```python
from build123d import *

# Parameters (mm, degrees)
SKETCH_1_W          = 60
SKETCH_1_H          = 31
EXTRUDE_1_DEPTH     = 10
CUT_EXTRUDE_1_DEPTH = 10
EXTRUDE_2_DEPTH     = 10
SKETCH_4_R          = 1
CUT_EXTRUDE_2_DEPTH = 10
SKETCH_5_W          = 39
SKETCH_5_H          = 20
SKETCH_5_W_2        = 0.67251462
SKETCH_5_H_2        = 5
SKETCH_5_W_3        = 11
SKETCH_5_H_3        = 2
CUT_EXTRUDE_3_DEPTH = 0.1
SKETCH_6_R          = 4
EXTRUDE_3_DEPTH     = 1.5
SKETCH_7_R          = 2
EXTRUDE_4_DEPTH     = 3


with BuildPart() as part:
    # 草图1 → 凸台-拉伸1 (new body)
    with BuildSketch(Plane(origin=(0, 0, 0), x_dir=(1, 0, 0), z_dir=(0, 1, 0))):
        with Locations((30, 15.5)):
            Rectangle(SKETCH_1_W, SKETCH_1_H)
    extrude(amount=EXTRUDE_1_DEPTH)

    # 草图2 → 切除-拉伸1 (cut)
    with BuildSketch(Plane(origin=(0, 10, 0), x_dir=(1, 0, 0), z_dir=(0, 1, 0))):
        Polygon((14, 0), (14, 1.5), (12.5, 1.5), (12.5, 3), (49.5, 3), (49.5, 2), (47, 2), (49.5, 0), align=None)
        Polygon((0, 30), (5, 31), (0, 31), align=None)
    extrude(amount=-CUT_EXTRUDE_1_DEPTH, mode=Mode.SUBTRACT)

    # 草图3 → 凸台-拉伸2 (add, through all)
    with BuildSketch(Plane(origin=(0, 10, 0), x_dir=(1, 0, 0), z_dir=(0, 1, 0))):
        with BuildLine():
            Line((61, 31), (60, 31))
            Line((60, 31), (60, 25))
            Line((60, 25), (61.7, 25))
            ThreePointArc((61.7, 25), (62.265685425, 25.234314575), (62.5, 25.8))
            Line((62.5, 25.8), (62.5, 28))
            Line((62.5, 28), (61, 31))
        make_face()
        Polygon((36, 31), (60, 31), (60, 32.5), (39.5, 32.5), align=None)
    extrude(amount=-EXTRUDE_2_DEPTH)

    # 草图4 → 切除-拉伸2 (cut)
    with BuildSketch(Plane.ZY):
        with Locations((-18.5, 5)):
            Circle(SKETCH_4_R)
        with Locations((-10.5, 5)):
            Circle(SKETCH_4_R)
    extrude(amount=-CUT_EXTRUDE_2_DEPTH, mode=Mode.SUBTRACT)

    # 草图5 → 切除-拉伸3 (cut)
    # profile 1 of 3: a face of its own
    with BuildSketch(Plane(origin=(0, 10, 0), x_dir=(1, 0, 0), z_dir=(0, 1, 0))):
        with Locations((34, 15)):
            Rectangle(SKETCH_5_W, SKETCH_5_H)
        Polygon((21.962260416, 17.792968637), (21.377465095, 17.792968637), (21.377465095, 21.360220099), (21.318985562, 21.360220099), (20.617231176, 17.792968637), (20.149394919, 17.792968637), (19.447640533, 21.360220099), (19.389161001, 21.360220099), (19.389161001, 17.792968637), (18.804365679, 17.792968637), (18.804365679, 22.792968637), (19.710798428, 22.792968637), (20.354073282, 19.48887507), (20.412552814, 19.48887507), (21.055827668, 22.792968637), (21.962260416, 22.792968637), align=None, mode=Mode.SUBTRACT)
        with Locations((24.111383223, 20.292968637)):
            Rectangle(SKETCH_5_W_2, SKETCH_5_H_2, mode=Mode.SUBTRACT)
        Polygon((29.359921235, 22.237413081), (28.190330592, 22.237413081), (28.190330592, 17.792968637), (27.517815972, 17.792968637), (27.517815972, 22.237413081), (26.348225329, 22.237413081), (26.348225329, 22.792968637), (29.359921235, 22.792968637), align=None, mode=Mode.SUBTRACT)
        with BuildLine():
            Line((33.102611293, 17.734489105), (32.60553527, 17.734489105))
            Line((32.60553527, 17.734489105), (32.517815972, 18.14384583))
            add(Edge.make_bspline(
                [(32.517815972, 18.14384583), (32.496335049, 18.114894908), (32.452578683, 18.05592225), (32.366892397, 17.979393037), (32.266643174, 17.909470256), (32.151128708, 17.848642528), (32.025699097, 17.798099411), (31.892521927, 17.760859691), (31.75360842, 17.739070297), (31.659108429, 17.736026374), (31.611383223, 17.734489105)],
                knots=[0, 0, 0, 0, 0.837184115, 1.705333332, 2.658671207, 3.677307666, 4.736711015, 5.80083511, 6.889358663, 8, 8, 8, 8], degree=3))
            add(Edge.make_bspline(
                [(31.611383223, 17.734489105), (31.560714868, 17.736021013), (31.46008263, 17.739063531), (31.311817937, 17.76762581), (31.16729555, 17.811965229), (31.027834691, 17.8755244), (30.891473719, 17.955281193), (30.760771836, 18.055054478), (30.632955326, 18.171046345), (30.509527994, 18.304333327), (30.396774962, 18.45853747), (30.297519239, 18.634098702), (30.215913122, 18.832381023), (30.147881926, 19.050856514), (30.096694353, 19.291330684), (30.05919444, 19.552513083), (30.036438806, 19.835379254), (30.033799786, 20.03103084), (30.032435855, 20.132149923)],
                knots=[0, 0, 0, 0, 0.758179789, 1.505818141, 2.253143624, 3.017869083, 3.795858856, 4.614441485, 5.475677495, 6.378750386, 7.330399785, 8.330312341, 9.391702904, 10.535751225, 11.753218739, 13.069914954, 14.485637047, 16, 16, 16, 16], degree=3))
            add(Edge.make_bspline(
                [(30.032435855, 20.132149923), (30.033524015, 20.243005064), (30.035631477, 20.457700531), (30.056303392, 20.768942629), (30.090571093, 21.058155718), (30.137547246, 21.32565553), (30.198737704, 21.571304744), (30.274571201, 21.795097166), (30.362412052, 21.997908599), (30.466184437, 22.177806713), (30.5809145, 22.336396595), (30.705728208, 22.474833232), (30.84257532, 22.589830475), (30.987256047, 22.687082934), (31.14384738, 22.76138369), (31.310614479, 22.812780351), (31.487019509, 22.845452192), (31.607987718, 22.849419101), (31.669862755, 22.851448169)],
                knots=[0, 0, 0, 0, 1.495213205, 2.895810661, 4.205263949, 5.422164245, 6.557127206, 7.616570214, 8.606403325, 9.533523062, 10.412081511, 11.242765381, 12.040838916, 12.817408929, 13.588463244, 14.369296309, 15.165897781, 16, 16, 16, 16], degree=3))
            add(Edge.make_bspline(
                [(31.669862755, 22.851448169), (31.724465447, 22.850157263), (31.831330219, 22.847630786), (31.986728106, 22.823055348), (32.133156944, 22.78417248), (32.270367528, 22.72996005), (32.39858198, 22.660001985), (32.517012997, 22.573895908), (32.626334766, 22.471986726), (32.725227795, 22.355220127), (32.813311094, 22.226144327), (32.892302084, 22.088427367), (32.956880517, 21.940329471), (33.009859712, 21.783333409), (33.052602879, 21.617693101), (33.080734277, 21.442188631), (33.100302009, 21.258143875), (33.101830982, 21.132132363), (33.102611293, 21.067822438)],
                knots=[0, 0, 0, 0, 1.017118894, 1.990637724, 2.924249984, 3.836374462, 4.733711419, 5.639510097, 6.558385009, 7.513001497, 8.485403533, 9.467718841, 10.467915617, 11.491402174, 12.553806325, 13.652248568, 14.801825996, 16, 16, 16, 16], degree=3))
            Line((33.102611293, 21.067822438), (32.45933644, 21.067822438))
            add(Edge.make_bspline(
                [(32.45933644, 21.067822438), (32.458729978, 21.117290953), (32.457551218, 21.213441346), (32.448009389, 21.352666796), (32.431312149, 21.482310098), (32.410867073, 21.602817265), (32.380914637, 21.71323506), (32.347227761, 21.814971363), (32.304498884, 21.905966508), (32.256760295, 21.988236327), (32.203036922, 22.060957155), (32.142500003, 22.123391188), (32.077558088, 22.176617179), (32.007055999, 22.22128447), (31.930094878, 22.254334745), (31.84783057, 22.277999378), (31.760739913, 22.29416845), (31.700622449, 22.295309026), (31.669862755, 22.295892614)],
                knots=[0, 0, 0, 0, 1.442265648, 2.803286258, 4.065667754, 5.252751118, 6.363271917, 7.39841691, 8.373155808, 9.288343585, 10.168233039, 11.001900497, 11.817228588, 12.611567034, 13.426963055, 14.24959516, 15.104388078, 16, 16, 16, 16], degree=3))
            add(Edge.make_bspline(
                [(31.669862755, 22.295892614), (31.631828893, 22.294563094), (31.557924625, 22.291979681), (31.450633434, 22.268061012), (31.350844775, 22.23047274), (31.257857421, 22.177333742), (31.172866818, 22.108722655), (31.097286108, 22.023210173), (31.025577535, 21.925676313), (30.964584262, 21.809804655), (30.908423102, 21.678016537), (30.863297772, 21.525387026), (30.821490016, 21.353610633), (30.790614597, 21.160102718), (30.763920798, 20.947080428), (30.748343708, 20.713136474), (30.735099548, 20.458990692), (30.734500993, 20.282340978), (30.734190241, 20.190629456)],
                knots=[0, 0, 0, 0, 0.713867664, 1.387128832, 2.054865043, 2.71116651, 3.391329963, 4.097256694, 4.850367561, 5.660840087, 6.551597142, 7.538616976, 8.647598492, 9.872123473, 11.218389466, 12.680914074, 14.276824714, 16, 16, 16, 16], degree=3))
            add(Edge.make_bspline(
                [(30.734190241, 20.190629456), (30.73483395, 20.103968299), (30.736071349, 19.937379816), (30.750607233, 19.698223249), (30.772176165, 19.47971091), (30.805076542, 19.282835127), (30.843512642, 19.105844287), (30.894744195, 18.950545195), (30.953134814, 18.815066175), (31.022715541, 18.70062504), (31.098039155, 18.604304965), (31.175512101, 18.520836306), (31.255451263, 18.450044406), (31.338684162, 18.392015675), (31.424300922, 18.345320992), (31.514153456, 18.314560623), (31.605733113, 18.293658802), (31.667942985, 18.291250783), (31.699102521, 18.29004466)],
                knots=[0, 0, 0, 0, 1.763137318, 3.38927359, 4.873732177, 6.228632264, 7.449226689, 8.554896297, 9.551299921, 10.444451664, 11.27164773, 12.035603122, 12.759076972, 13.439665674, 14.096862192, 14.735741838, 15.366761318, 16, 16, 16, 16], degree=3))
            add(Edge.make_bspline(
                [(31.699102521, 18.29004466), (31.72983218, 18.290848844), (31.790132284, 18.292426876), (31.878031693, 18.305615952), (31.961197096, 18.327367151), (32.039477559, 18.357607005), (32.112590811, 18.396886673), (32.180290182, 18.444875026), (32.24233728, 18.502053953), (32.300237525, 18.567322721), (32.352177249, 18.64200929), (32.396916088, 18.726819825), (32.434506327, 18.820857568), (32.464574283, 18.924703583), (32.488267476, 19.037669605), (32.505105864, 19.159978961), (32.516471005, 19.291925027), (32.517356401, 19.383080592), (32.517815972, 19.430395538)],
                knots=[0, 0, 0, 0, 0.926763241, 1.818566216, 2.674466499, 3.515830513, 4.344194496, 5.172200422, 6.012506428, 6.88440238, 7.799833367, 8.749917039, 9.771239203, 10.849892544, 12.007626437, 13.250589984, 14.572899121, 16, 16, 16, 16], degree=3))
            Line((32.517815972, 19.430395538), (32.517815972, 19.752032964))
            Line((32.517815972, 19.752032964), (31.611383223, 19.752032964))
            Line((31.611383223, 19.752032964), (31.611383223, 20.30758852))
            Line((31.611383223, 20.30758852), (33.102611293, 20.30758852))
            Line((33.102611293, 20.30758852), (33.102611293, 17.734489105))
        make_face(mode=Mode.SUBTRACT)
    # profile 2 of 3: a face of its own
    with BuildSketch(Plane(origin=(0, 10, 0), x_dir=(1, 0, 0), z_dir=(0, 1, 0))):
        with Locations((6.5, 18.646769807)):
            Rectangle(SKETCH_5_W_3, SKETCH_5_H_3)
        Polygon((3.383335667, 18.64715665), (2.749062348, 18.08056229), (2.749062348, 18.460605674), (1.671405081, 18.460605674), (1.671405081, 18.851495045), (2.749062348, 18.851495045), (2.749062348, 19.245855132), align=None, mode=Mode.SUBTRACT)
    # profile 3 of 3: a face of its own
    with BuildSketch(Plane(origin=(0, 10, 0), x_dir=(1, 0, 0), z_dir=(0, 1, 0))):
        with Locations((6.5, 10.646769807)):
            Rectangle(SKETCH_5_W_3, SKETCH_5_H_3)
        Polygon((3.551150659, 10.362171108), (2.473927231, 10.362171108), (2.473927231, 9.979524687), (1.834013999, 10.563038787), (2.473927231, 11.138743776), (2.473927231, 10.753060479), (3.551150659, 10.753060479), align=None, mode=Mode.SUBTRACT)
    extrude(amount=-CUT_EXTRUDE_3_DEPTH, mode=Mode.SUBTRACT)

    # 草图6 → 凸台-拉伸3 (add)
    with BuildSketch(Plane(origin=(60, 0, 0), x_dir=(0, 0, -1), z_dir=(1, 0, 0))):
        with Locations(Location((11, 5, 0), (0, 0, 180))):
            Circle(SKETCH_6_R)
    extrude(amount=EXTRUDE_3_DEPTH)

    # 草图7 → 凸台-拉伸4 (add)
    with BuildSketch(Plane(origin=(61.5, 0, 0), x_dir=(0, 0, -1), z_dir=(1, 0, 0))):
        with Locations((11, 5)):
            Circle(SKETCH_7_R)
    extrude(amount=EXTRUDE_4_DEPTH)


solid = part.part
```
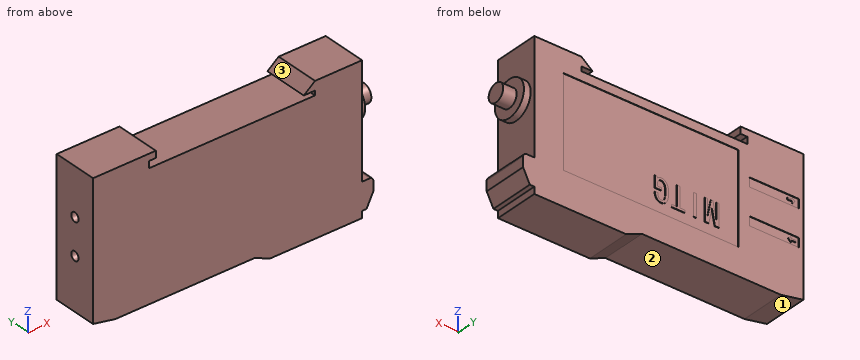
The listing builds one solid part. Answer for the finished solid, in the listing's coordinates (mm). Face numbers are marked on the shaded views. Give positions to 0.01 mm unless a question says otherwise; leave off trailing zeros. Order: outer loops, then holes, each group sorted by start corner. A loop starts at its lowest first (then second) coordinate and runs counter-clockwise, first axis right, second up. Notation, with made-up numbers: (26.5, -26.5) - (77.5, -26.5) arc R20 cw to (77.5, 5.5) - close; hole circle Ø10 at (-11, -18.75). An arc over 180 degrees is marked (long way). Answer in a Markdown table with one row per item. Add a question column.
Q1. Find the intervals of material crossed by line 1 along Y through (x, z) = (7.25, -10.5); line 2 along Z through (x, y) = (20, 9); line 3 along X through (y, z) = (8, -22.5), in increasing order. Write a range as [from, to].
Q2. For a pull along X with two mould halves and no side action, classify the marked faces 1, 2 and 3 as released by +X, released by -X, zero draft, split by the parting line, or undercut.
Q3. The part is cut by section C-C (x = 46). Determine the outline of the cut face in (y, z), then the cut area to 3 significant figures.
Q4. Given P1, Ø0.8, axis at y = 6.5, z = -2, coming from the +X side; P2, Ø3, axis at y = 1, z = -27, coming from the +X side; P3, Ø3, axis at x = 51, z = -21.5, coming from the +Y side, each flat-ended and moving along its own axis, determine where each tip first touches the part or whether it passes through.
Q5. The part is cut by section A-A (x = 6). Determine the outline of the cut face in (y, z), then the cut area to 3 significant figures.
Q6. The part is cut by section B-B (z = -8). Determine the outline of the cut face in (x, y).
Determined:
| question | item | result |
|---|---|---|
| 1 | line 1 | y = [0, 4], [6, 9.9] |
| 1 | line 2 | z = [-31, -3] |
| 1 | line 3 | x = [0, 60] |
| 2 | face 1 | released by -X |
| 2 | face 2 | zero draft |
| 2 | face 3 | undercut |
| 3 | outline | (0, -32.5) - (10, -32.5) - (10, -25) - (9.9, -25) - (9.9, -5) - (10, -5) - (10, -3) - (0, -3) - close |
| 3 | area | 293 mm² |
| 4 | P1 | stops at x = 60 |
| 4 | P2 | stops at x = 62.5 |
| 4 | P3 | stops at y = 9.9 |
| 5 | outline | (0, -31) - (10, -31) - (10, -19.65) - (9.9, -19.65) - (9.9, -17.65) - (10, -17.65) - (10, -11.65) - (9.9, -11.65) - (9.9, -9.65) - (10, -9.65) - (10, 0) - (0, 0) - close; hole circle Ø2 at (5, -18.5); hole circle Ø2 at (5, -10.5) |
| 5 | area | 303 mm² |
| 6 | outline | (0, 0) - (60, 0) - (60, 2.35) - (61.5, 2.35) - (61.5, 7.65) - (60, 7.65) - (60, 10) - (53.5, 10) - (53.5, 9.9) - (14.5, 9.9) - (14.5, 10) - (0, 10) - close |
